```python
from build123d import *

# Parameters (mm, degrees)
SKETCH1_W           = 40
SKETCH1_H           = 40
BOSS_EXTRUDE1_DEPTH = 27.6
CUT_EXTRUDE1_DEPTH  = 41
SKETCH3_R           = 2.5
CUT_EXTRUDE2_DEPTH  = 14.6
CHAMFER1_SIZE       = 1.5


with BuildPart() as part:
    # Sketch1 → Boss-Extrude1 (new body)
    with BuildSketch(Plane(origin=(0, 0, 0), x_dir=(1, 0, 0), z_dir=(0, 1, 0))):
        Rectangle(SKETCH1_W, SKETCH1_H)
    extrude(amount=BOSS_EXTRUDE1_DEPTH)

    # Sketch2 → Cut-Extrude1 (cut, through all)
    with BuildSketch(Plane.XY.offset(20)):
        with BuildLine():
            Line((9.141218295, 0), (-9.141218295, 0))
            Line((-9.141218295, 0), (-3.619707233, 7.772105397))
            ThreePointArc((-3.619707233, 7.772105397), (0, 19.117222623), (3.619707233, 7.772105397))
            Line((3.619707233, 7.772105397), (9.141218295, 0))
        make_face()
    extrude(amount=-CUT_EXTRUDE1_DEPTH, mode=Mode.SUBTRACT)

    # Sketch3 → Cut-Extrude2 (cut)
    with BuildSketch(Plane(origin=(0, 27.6, 0), x_dir=(1, 0, 0), z_dir=(0, 1, 0))):
        with Locations((-14, 13)):
            Circle(SKETCH3_R)
        with Locations((14, 13)):
            Circle(SKETCH3_R)
        with Locations((14, -13)):
            Circle(SKETCH3_R)
        with Locations((-14, -13)):
            Circle(SKETCH3_R)
    extrude(amount=-CUT_EXTRUDE2_DEPTH, mode=Mode.SUBTRACT)

    # Chamfer1
    chamfer1_edges = [part.edges().sort_by_distance(p)[0] for p in [
        (-20, 27.6, 0),
        (20, 27.6, 0),
        (-20, 0, 0),
        (20, 0, 0),
    ]]
    chamfer(chamfer1_edges, length=CHAMFER1_SIZE)


solid = part.part
```
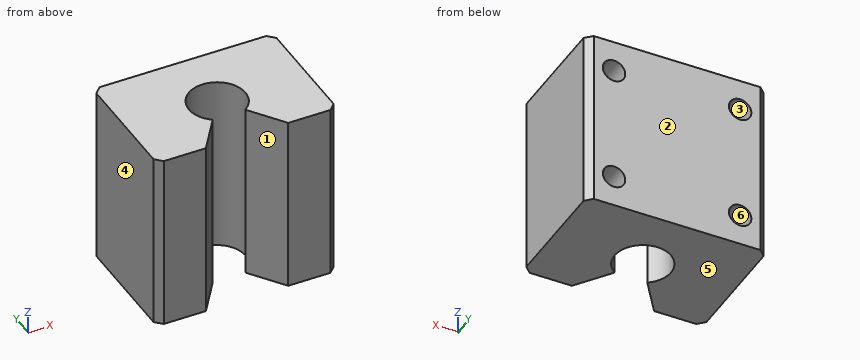
For this review, take the finished solid that the model builds, in its own axes (mm). Face numbers are marked on the shaded views. A direction names the side the tool comes from. Round coordinates to 2 decimals unless told otherwise and drop trailing zeros. Order: outer loops, then holes, each group sorted by start corner. A loop starts at its lowest first (then second) coordinate and runs counter-clockwise, first axis right, second up.
Q1. Insertion check: P1, Ø4, axis at x = 14, z = -13, coming from the +Y side; P2, Ø6.5, axis at x = -14, z = 13, coming from the +Y side; P3, Ø7.5, axis at x = 0, y = 12.87, coming from the -Z side. Each pin has a flat end and moves straight along its axis. Give the tip position at first contact, or say it passes through.
Findings below:
P1: stops at y = 13
P2: stops at y = 27.6
P3: passes through
Q2. Wall thickness on line 1 (Z direction, x = -14, y = 15.25); line 2 (X direction, y = 21.25, z = -13); line 3 (X direction, y = 18, z = 13): over which ranges is each line inside the solid? List them lowest first.
Findings below:
line 1: z = -20 to -15.5, -10.5 to 10.5, 15.5 to 20
line 2: x = -20 to -16.5, -11.5 to 11.5, 16.5 to 20
line 3: x = -20 to -16.5, -11.5 to -3.57, 3.57 to 11.5, 16.5 to 20
Q3. We need section C-C, the plane z = 13. Give the boundary of the cut face in (x, y), plus the area to 3 significant figures.
Findings below:
outline: (-20, 1.5) - (-18.5, 0) - (-9.14, 0) - (-3.62, 7.77) arc R6.25 cw (long way) to (3.62, 7.77) - (9.14, 0) - (18.5, 0) - (20, 1.5) - (20, 26.1) - (18.5, 27.6) - (16.5, 27.6) - (16.5, 13) - (11.5, 13) - (11.5, 27.6) - (-11.5, 27.6) - (-11.5, 13) - (-16.5, 13) - (-16.5, 27.6) - (-18.5, 27.6) - (-20, 26.1) - close
area: 737 mm2
Q4. Machinability: for the marked faces 1, 2 and 3, which of the approach directions +Z, -Z, +X, -X, +Y, -Y give a long, thin tool a straight path to every point of the face, cutting with its end or side? Answer none if there is none.
Findings below:
face 1: +Z, -Z, -Y
face 2: +Z, -Z, +X, -X, +Y
face 3: +Y
Q5. We need section D-D, the plane y = 10.25. Give the boundary of the cut face in (x, z).
Findings below:
outline: (-20, -20) - (-5.68, -20) - (-5.68, 20) - (-20, 20) - close; (5.68, -20) - (20, -20) - (20, 20) - (5.68, 20) - close
Q6. We need section A-A, the plane y = 23. Give the boundary of the cut face in (x, z), plus the area to 3 significant figures.
Findings below:
outline: (-20, -20) - (20, -20) - (20, 20) - (-20, 20) - close; hole circle Ø5 at (-14, -13); hole circle Ø5 at (-14, 13); hole circle Ø5 at (14, -13); hole circle Ø5 at (14, 13)
area: 1,520 mm2
Q7. We need section B-B, the plane x = -14. Give the boundary of the cut face in (y, z), plus the area to 3 significant figures.
Findings below:
outline: (0, -20) - (27.6, -20) - (27.6, -15.5) - (13, -15.5) - (13, -10.5) - (27.6, -10.5) - (27.6, 10.5) - (13, 10.5) - (13, 15.5) - (27.6, 15.5) - (27.6, 20) - (0, 20) - close
area: 958 mm2
Q8. Mouldability with a two-part tool opening along X and no side actions: class the marked faces 4, 5 and 6 as pulls with the +X half, pulls with the -X half, needs draft (parallel to the pull), parting line crosses it, or undercut.
Findings below:
face 4: pulls with the -X half
face 5: needs draft
face 6: undercut
